```python
from build123d import *

# Parameters (mm, degrees)
SKETCH_1_R          = 3.5
EXTRUDE_1_DEPTH     = 5
SKETCH_2_R          = 2.25
EXTRUDE_2_DEPTH     = 3
CHAMFER_1_SIZE      = 0.2
SKETCH_4_R          = 1.25
CUT_EXTRUDE_1_DEPTH = 9
CHAMFER_2_SIZE      = 0.2


with BuildPart() as part:
    # Эскиз1 → Бобышка-Вытянуть1 (new body)
    with BuildSketch(Plane.XY):
        Circle(SKETCH_1_R)
    extrude(amount=EXTRUDE_1_DEPTH)

    # Эскиз2 → Бобышка-Вытянуть2 (add)
    with BuildSketch(Plane(origin=(0, 0, 0), x_dir=(-1, 0, 0), z_dir=(0, 0, -1))):
        with Locations(Location((0, 0, 0), (0, 0, 180))):
            Circle(SKETCH_2_R)
    extrude(amount=EXTRUDE_2_DEPTH)

    # Фаска1
    chamfer_1_edges = [part.edges().sort_by_distance(p)[0] for p in [
        (-3.5, 0, 0),
        (-3.5, 0, 5),
        (-2.25, 0, -3),
    ]]
    chamfer(chamfer_1_edges, length=CHAMFER_1_SIZE)

    # Эскиз4 → Вырез-Вытянуть1 (cut)
    with BuildSketch(Plane.XY.offset(5)):
        Circle(SKETCH_4_R)
    extrude(amount=-CUT_EXTRUDE_1_DEPTH, mode=Mode.SUBTRACT)

    # Фаска2
    chamfer_2_edges = [part.edges().sort_by_distance(p)[0] for p in [
        (-1.25, 0, -3),
        (-1.25, 0, 5),
    ]]
    chamfer(chamfer_2_edges, length=CHAMFER_2_SIZE)


solid = part.part
```
Could you check a few things on this model? Use its own coordinates, in mm. A direction names the side the tool comes from. Coordinates: 2 decimals unless noted, no trailing zeros. Write each loop counter-clockwise with the first axis right and the second up, starting at its lowest first coordinate (ties: lowest second). Pieces come first, ordered by that corner, then holes. Notation, with made-up numbers: (-28.75, 33.5) -> (-7.75, 33.5) arc R32 ccw to (-7.75, 70.5) -> close; hole circle Ø4 at (4, -32). An arc over 180 degrees is marked (long way). One line per question, with ' | ' between items. Start each with the question number.
1. For faces 4 (the face through (-1.66, -1.52, -1.38)), 5 (the face through (0.88, 1.34, -3)), which set-ups out of +Z, -Z, +X, -X, +Y, -Y let a thin tool reach every point of the face, with its end or its side?
2. If we section it at D-D (z = -0.5): Please give me the cut outline in (x, y), and give its area (3 significant figures).
3. If we section it at C-C (z = 2.5): Please give me the cut outline in (x, y), and give its area (3 significant figures).
4. If we section it at A-A (y = 0): Please give me the cut outline in (x, z), and give its area (3 significant figures).
5. Please list where these lines run through material, in increasing order: line 1 along Y through (x, z) = (0, 1.75); line 2 along Y through (x, z) = (0, -1); line 3 along Z through (x, y) = (-1.5, -1.75).
6. Will this pin go through, and if not, where does the flat tip stop? P1, Ø2, axis at y = -1.5, z = 2, coming from the +X side.
7. Thinking about a two-plate mould opening in Y: for faces 1 (the face through (3.233, -1.341, 2.468)), 2 (the face through (-0.27, -1.22, 1.05)), 3 (the face through (1.4, -2.2, 0)), which applies, pulls with the +Y half, pulls with the -Y half, needs draft (parallel to the pull), parting line crosses it, or undercut?
Return value:
1) face 4: -Z | face 5: -Z, +X, -X, +Y, -Y
2) outline: circle Ø4.5 at (0, 0); hole circle Ø2.5 at (0, 0) | area: 11.0 mm²
3) outline: circle Ø7 at (0, 0); hole circle Ø2.5 at (0, 0) | area: 33.6 mm²
4) outline: (-3.5, 0.2) -> (-3.3, 0) -> (-2.25, 0) -> (-2.25, -2.8) -> (-2.05, -3) -> (-1.45, -3) -> (-1.25, -2.8) -> (-1.25, 4.8) -> (-1.45, 5) -> (-3.3, 5) -> (-3.5, 4.8) -> close; (1.25, -2.8) -> (1.45, -3) -> (2.05, -3) -> (2.25, -2.8) -> (2.25, 0) -> (3.3, 0) -> (3.5, 0.2) -> (3.5, 4.8) -> (3.3, 5) -> (1.45, 5) -> (1.25, 4.8) -> close | area: 28.3 mm²
5) line 1: y = -3.5 to -1.25, 1.25 to 3.5 | line 2: y = -2.25 to -1.25, 1.25 to 2.25 | line 3: z = 0 to 5
6) P1: stops at x = 3.46
7) face 1: parting line crosses it | face 2: undercut | face 3: needs draft
